Autodesk Inventor part; units mm, degrees
ref_plane "YZ Plane" through (0, 0, 0) normal (1, 0, 0) x (0, 1, 0)
ref_plane "XZ Plane" through (0, 0, 0) normal (0, 1, 0) x (-1, 0, 0)
ref_plane "XY Plane" through (0, 0, 0) normal (0, 0, 1) x (1, 0, 0)
sketch "Sketch1" plane through (0, 0, 0) normal (0, 0, 1) x (1, 0, 0)
  line L0 (-21.1557, 36.079) -> (-21.1557, -5.831)
  line L1 (-21.1557, -5.831) -> (-2.1057, -5.831)
  line L2 (-2.1057, -5.831) -> (-2.1057, 36.079)
  line L3 (-2.1057, 36.079) -> (-5.2807, 36.079)
  line L4 (-5.2807, 36.079) -> (-5.2807, 17.029)
  line L5 (-5.2807, 17.029) -> (-17.9807, 17.029)
  line L6 (-17.9807, 17.029) -> (-17.9807, 36.079)
  line L7 (-17.9807, 36.079) -> (-21.1557, 36.079)
  point P0 (0, 0)
  dimension "d0" = 19.05
  dimension "d1" = 12.7
  dimension "d2" = 3.175
  dimension "d3" = 3.175
  dimension "d4" = 41.91
  dimension "d5" = 19.05
  dimension "d6" = 0
extrude "Extrusion1" add sketch "Sketch1" along normal blind 19.05
sketch "Sketch2" plane through (-21.1557, -5.831, 0) normal (0, -1, 0) x (1, 0, 0)
  circle A0 centre (9.525, 9.525) radius 6.35
  point P0 (21.1557, 0)
  dimension "d9" = 12.7
extrude "Extrusion2" cut sketch "Sketch2" against normal blind 21.59
sketch "Sketch3" plane through (-21.1557, -5.831, 0) normal (-1, 0, 0) x (0, 0, 1)
  line L0 (0, 41.91) -> (19.05, 41.91)
  circle A0 centre (9.525, 33.02) radius 4.7625
  point P0 (0, 5.831)
  dimension "d12" = 9.525
  dimension "d13" = 8.89
extrude "Extrusion3" cut sketch "Sketch3" against normal through all
thread "Thread1"
properties part number "1in Actuator Clovis 1764"
Here's how the part is built. I have some questions about the finished solid (model axes, mm). A direction names the side the tool comes from. Coordinates: 2 decimals unless noted, no trailing zeros. Order: outer loops, then holes, each group sorted by start corner. A loop starts at its lowest first (then second) coordinate and runs counter-clockwise, first axis right, second up. Notation, with made-up numbers: (17.25, 60) - (35.25, 60) arc R19 cw to (35.25, 89) - close; hole circle Ø11 at (72, 26.25). An arc over 180 degrees is marked (long way). One line per question, with ' | ' between items.
(1) If I drill on L1, parallel to X at y = 22.5, z = 2.25; L2, parallel to Y at x = -19, z = 9.5; L3, parallel to Z at x = -11.5, y = 12, over which ranges is the centre line in solid material (lowest first)?
Report:
L1: x = -21.16 to -17.98, -5.28 to -2.11 | L2: y = -5.83 to 22.43, 31.95 to 36.08 | L3: z = 0 to 3.18, 15.87 to 19.05
(2) Suppose I cut it at A-A on z = 10.5. List the corners of the cut face in (x, y) for me, and give its area (3 significant figures).
Report:
outline: (-21.16, -5.83) - (-17.91, -5.83) - (-17.91, 15.76) - (-5.36, 15.76) - (-5.36, -5.83) - (-2.11, -5.83) - (-2.11, 22.53) - (-5.28, 22.53) - (-5.28, 17.03) - (-17.98, 17.03) - (-17.98, 22.53) - (-21.16, 22.53) - close; (-21.16, 31.85) - (-17.98, 31.85) - (-17.98, 36.08) - (-21.16, 36.08) - close; (-5.28, 31.85) - (-2.11, 31.85) - (-2.11, 36.08) - (-5.28, 36.08) - close | area: 226 mm2
(3) Will these pins go through, and if not, where does the flat tip stop? pin 1 (4 mm diameter, centred on x = -8.5, z = 11, fed in from -Y); pin 2 (10 mm diameter, centred on x = -10.5, z = 13.5, fed in from +Y).
Report:
pin 1: stops at y = 15.76 | pin 2: stops at y = 17.03
(4) Suppose I cut it at D-D on z = 17.5. List the corners of the cut face in (x, y) for me, and give its area (3 significant figures).
Report:
outline: (-21.16, -5.83) - (-2.11, -5.83) - (-2.11, 36.08) - (-5.28, 36.08) - (-5.28, 17.03) - (-17.98, 17.03) - (-17.98, 36.08) - (-21.16, 36.08) - close | area: 556 mm2
(5) Suppose I cut it at C-C on x = -6.5. List the corners of the cut face in (y, z) for me, and give its area (3 significant figures).
Report:
outline: (-5.83, 0) - (17.03, 0) - (17.03, 19.05) - (-5.83, 19.05) - (-5.83, 13.27) - (15.76, 13.27) - (15.76, 5.78) - (-5.83, 5.78) - close | area: 274 mm2
(6) Suppose I cut it at B-B on y = 30. List the corners of the cut face in (x, z) for me, and give its area (3 significant figures).
Report:
outline: (-21.16, 0) - (-17.98, 0) - (-17.98, 5.68) - (-21.16, 5.68) - close; (-21.16, 13.37) - (-17.98, 13.37) - (-17.98, 19.05) - (-21.16, 19.05) - close; (-5.28, 0) - (-2.11, 0) - (-2.11, 5.68) - (-5.28, 5.68) - close; (-5.28, 13.37) - (-2.11, 13.37) - (-2.11, 19.05) - (-5.28, 19.05) - close | area: 72.1 mm2
(7) If we mould it in two halves opening along Z, with no side actions, what happens to faces 4 (the flat face through (-12, 11, 19.05)), 5 (the cylindrical face through (-19.59, 22.54, 8.49)), 6 (the cylindrical face through (-13.007, 4.813, 3.326)), 7 (the flat face through (-4, 36.079, 9))? For each: pulls with the +Z half, pulls with the -Z half, needs draft (parallel to the pull), parting line crosses it, or undercut.
Report:
face 4: pulls with the +Z half | face 5: undercut | face 6: undercut | face 7: needs draft
(8) For faces 1 (the flat face through (-2.106, 15, 9)), 2 (the flat face through (-12, 15.759, 10)), 3 (the flat face through (-5.281, 22, 12)), which set-ups out of +Z, -Z, +X, -X, +Y, -Y let a thin tool reach every point of the face, with its end or its side?
Report:
face 1: +Z, -Z, +X, +Y, -Y | face 2: -Y | face 3: +Z, -Z, +Y
